The drawing under review shows one solid part. Ordinate dimensions are in mm from its lowest x, y, z. A direction names the side the tool comes from. Coordinates: 2 decimals unless noted, no trailing zeros. Loops run counter-clockwise (first coordinate to the right, second up) from the corner with the lowest first, then second, coordinate; pieces in that order, holes last. Notation, with made-up numbers: M 65.25,75 L 72.25,75 A26 cw 72.25,107 Z; hole C 85.5,85 d6. An arc over 180 degrees is marked long. Put each result on its own line as item: value.
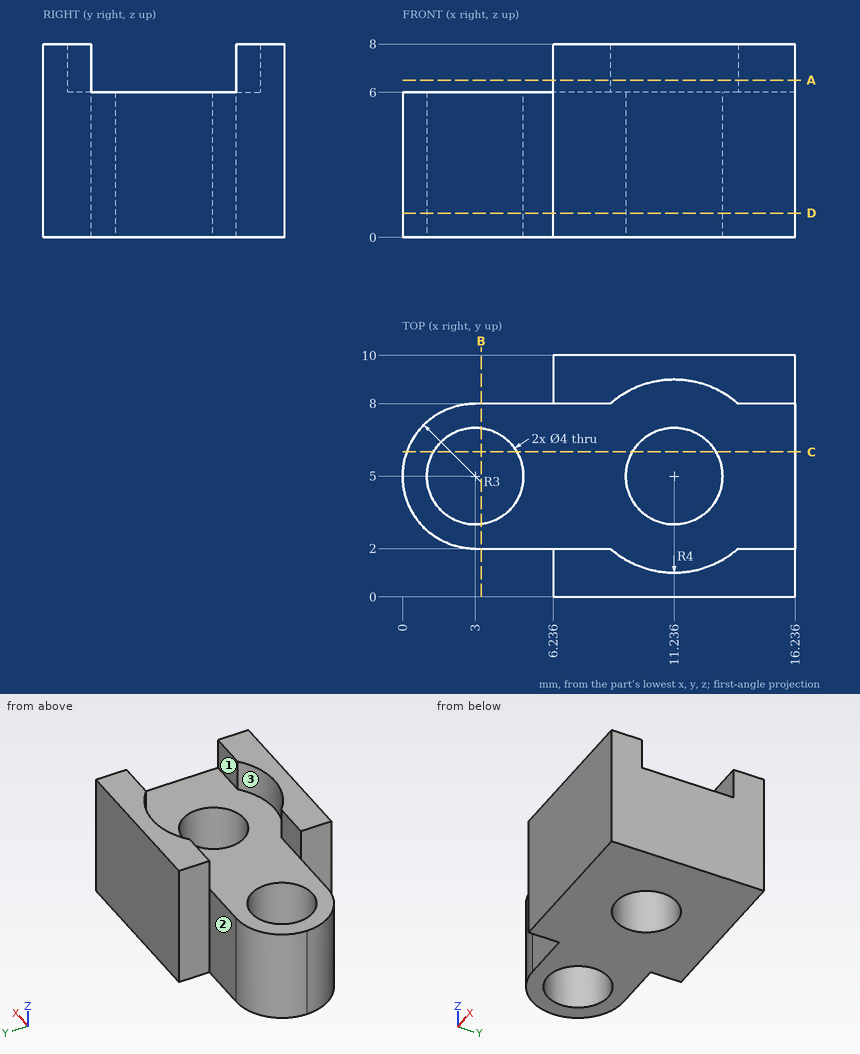
(1) Tool access review of the marked faces 1, 2 and 3: name each direction out of +Z, -Z, +X, -X, +Y, -Y from which nothing blocks a thin tool from reaching the whole face with its end or side.
Determined:
face 1: +Z, +X, -X
face 2: +Z, -Z, -X, +Y
face 3: +Z
(2) Wall thickness on line 1 along X through (y, z) = (5, 3.2) (1 decimal); line 2 along X through (y, z) = (5.75, 5) (1 decimal); line 3 along Z through (x, y) = (15.75, 4.5): over which ranges is each line inside the solid? List them lowest first. Write a range as [from, to].
Determined:
line 1: x = [0, 1], [5, 9.2], [13.2, 16.2]
line 2: x = [0.1, 1.1], [4.9, 9.4], [13.1, 16.2]
line 3: z = [0, 6]
(3) Add section D-D (z = 1). Write out the cut boundary in (x, y) (1 decimal).
Determined:
outline: M 3,2 L 6.2,2 L 6.2,0 L 16.2,0 L 16.2,10 L 6.2,10 L 6.2,8 L 3,8 A3 ccw Z; hole C 3,5 d4; hole C 11.2,5 d4
(4) For pin 1 (4 mm diameter, centred on x = 2.5, y = 5, fed in from +Z); pin 2 (1.6 mm diameter, centred on x = 4.5, z = 4, fed in from +Y); pin 3 (0.6 mm diameter, centred on y = 1.5, z = 2, fed in from -X), all flat-tipped, find the tip position at first contact; note any pin that passes through.
Determined:
pin 1: stops at z = 6
pin 2: stops at y = 8
pin 3: stops at x = 6.24
(5) Add section A-A (z = 6.5). Write out the cut boundary in (x, y) (1 decimal).
Determined:
outline: M 6.2,0 L 16.2,0 L 16.2,2 L 13.9,2 A4 cw 8.6,2 L 6.2,2 Z; M 6.2,8 L 8.6,8 A4 cw 13.9,8 L 16.2,8 L 16.2,10 L 6.2,10 Z
(6) Add section C-C (y = 6). Write out the cut boundary in (x, z) (1 decimal).
Determined:
outline: M 0.2,0 L 1.3,0 L 1.3,6 L 0.2,6 Z; M 4.7,0 L 9.5,0 L 9.5,6 L 4.7,6 Z; M 13,0 L 16.2,0 L 16.2,6 L 13,6 Z
(7) Add section B-B (x = 3.25). Write out the cut boundary in (y, z) (1 decimal), plus the area to 3 significant figures.
Determined:
outline: M 2,0 L 3,0 L 3,6 L 2,6 Z; M 7,0 L 8,0 L 8,6 L 7,6 Z
area: 12.2 mm^2
